from build123d import *

# Parameters (mm, degrees)
SKETCH1_R           = 107.09
BOSS_EXTRUDE1_DEPTH = 3
CUT_EXTRUDE1_START  = -3
CUT_EXTRUDE1_DEPTH  = 4
CIRPATTERN1_COUNT   = 8
SKETCH7_W           = 3
SKETCH7_H           = 5
CUT_EXTRUDE4_DEPTH  = 3
CIRPATTERN2_COUNT   = 8
SKETCH4_R           = 1.5
SKETCH4_W           = 66
SKETCH4_H           = 30
CUT_EXTRUDE5_DEPTH  = 10
CUT_EXTRUDE6_DEPTH  = 3


with BuildPart() as part:
    # Sketch1 → Boss-Extrude1 (new body)
    with BuildSketch(Plane(origin=(0, 0, 0), x_dir=(1, 0, 0), z_dir=(0, 1, 0))):
        Circle(SKETCH1_R)
    extrude(amount=BOSS_EXTRUDE1_DEPTH)

    # Sketch2 → Cut-Extrude1 (cut)
    with BuildSketch(Plane(origin=(0, 3, 0), x_dir=(1, 0, 0), z_dir=(0, 1, 0)).offset(CUT_EXTRUDE1_START)):
        Polygon((-1.5, 597.330930071), (-1.5, 107.079494302), (-1.5, 97.079494302), (1.5, 97.079494302), (1.5, 107.079494302), (1.5, 597.330930071), (1.5, 1577.83380161), (-1.5, 1577.83380161), align=None)
    cut_extrude1 = extrude(amount=CUT_EXTRUDE1_DEPTH, mode=Mode.SUBTRACT)

    # CirPattern1: Cut-Extrude1 ×8 about axis
    cirpattern1_axis = Axis((0, 0, 0), (0, -1, 0))
    for i in range(1, CIRPATTERN1_COUNT):
        add(cut_extrude1.rotate(cirpattern1_axis, i * 360 / CIRPATTERN1_COUNT), mode=Mode.SUBTRACT)

    # Sketch7 → Cut-Extrude4 (cut)
    with BuildSketch(Plane(origin=(0, 3, 0), x_dir=(1, 0, 0), z_dir=(0, 1, 0))):
        with Locations((-3.5, 93.579494302)):
            Rectangle(SKETCH7_W, SKETCH7_H)
        with Locations((3.5, 93.579494302)):
            Rectangle(SKETCH7_W, SKETCH7_H)
    cut_extrude4 = extrude(amount=-CUT_EXTRUDE4_DEPTH, mode=Mode.SUBTRACT)

    # CirPattern2: Cut-Extrude4 ×8 about axis
    cirpattern2_axis = Axis((0, 0, 0), (0, 1, 0))
    for i in range(1, CIRPATTERN2_COUNT):
        add(cut_extrude4.rotate(cirpattern2_axis, i * 360 / CIRPATTERN2_COUNT), mode=Mode.SUBTRACT)

    # Sketch4 → Cut-Extrude5 (cut)
    with BuildSketch(Plane(origin=(0, 3, 0), x_dir=(1, 0, 0), z_dir=(0, 1, 0))):
        with Locations((-57, 9.5)):
            Circle(SKETCH4_R)
        with Locations((-57, -9.5)):
            Circle(SKETCH4_R)
        with Locations((21, -9.5)):
            Circle(SKETCH4_R)
        with Locations((21, 9.5)):
            Circle(SKETCH4_R)
        with Locations((-18, 0)):
            Rectangle(SKETCH4_W, SKETCH4_H)
        with BuildLine():
            Line((72.75038213, -25.5), (-72.75038213, -25.5))
            ThreePointArc((-72.75038213, -25.5), (0, -77.09), (72.75038213, -25.5))
        make_face()
        with BuildLine():
            Line((72.75038213, 25.5), (-72.75038213, 25.5))
            ThreePointArc((-72.75038213, 25.5), (0, 77.09), (72.75038213, 25.5))
        make_face()
    extrude(amount=-CUT_EXTRUDE5_DEPTH, mode=Mode.SUBTRACT)

    # Sketch9 → Cut-Extrude6 (cut)
    with BuildSketch(Plane(origin=(0, 3, 0), x_dir=(1, 0, 0), z_dir=(0, 1, 0))):
        Polygon((-35.879388071, -94.459883081), (-33.107749474, -95.607933378), (-26.219447691, -78.978101793), (-28.991086289, -77.830051496), align=None)
        Polygon((-19.249556486, -101.348184863), (-16.477917889, -102.49623516), (-9.589616106, -85.866403575), (-12.361254704, -84.718353278), align=None)
        Polygon((53.935833667, 67.497598822), (60.824135449, 84.127430407), (58.052496852, 85.275480704), (51.164195069, 68.645649119), align=None)
        Polygon((37.306002081, 74.385900604), (44.194303864, 91.015732189), (41.422665266, 92.163782487), (34.534363484, 75.533950901), align=None)
    extrude(amount=-CUT_EXTRUDE6_DEPTH, mode=Mode.SUBTRACT)


solid = part.part
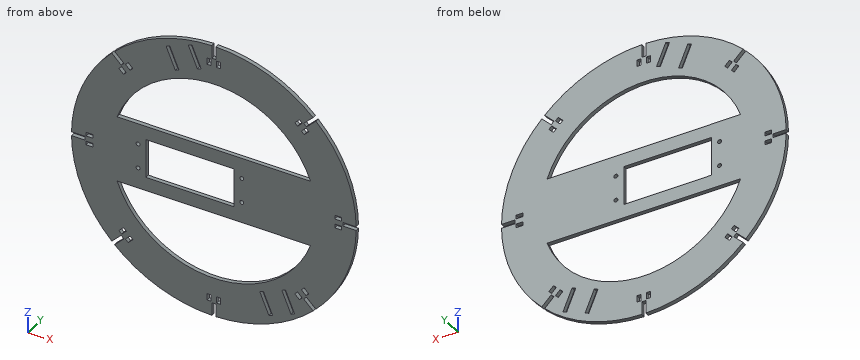
Could you check a few things on this model? Use its own coordinates, in mm. Coordinates: 2 decimals unless noted, no trailing zeros. Write each loop counter-clockwise with the first axis right and the second up, starting at its lowest first coordinate (ties: lowest second). Pieces come first, ordered by that corner, then holes. Notation, with made-up numbers: (74.5, 74.25) - (93.5, 74.25) arc R24 cw to (93.5, 90.25) - close; hole circle Ø9 at (30.5, 25). An arc over 180 degrees is marked (long way). Write item = value, one per line.
1) Suppose I cut it at A-A on x = 48. Please give me the cut outline in (y, z), plus the area to 3 significant figures.
Result set:
outline = (0, -95.73) - (3, -95.73) - (3, -60.32) - (0, -60.32) - close; (0, -25.5) - (3, -25.5) - (3, 25.5) - (0, 25.5) - close; (0, 60.32) - (3, 60.32) - (3, 95.73) - (0, 95.73) - close
area = 365 mm2
2) Suppose I cut it at C-C on y = 2.4. State how many separate pieces and enclosed holes the cut face has, plus the area to 3 significant figures.
Result set:
separate_pieces = 1
enclosed_holes = 27
area = 22,400 mm2
3) Please list where these lines run through material, in increasing order: line 1 (X direction, y = 1.2, z = 4.5); line 2 (Z direction, x = -33.5, y = 0.65); line 3 (X direction, y = 2.25, z = 68.5). Write a range as [from, to].
Result set:
line_1 = [-107, -96.08], [-91.08, -51], [15, 91.08], [96.08, 107]
line_2 = [-101.72, -69.43], [-25.5, -15], [15, 25.5], [69.43, 88.72], [95.45, 101.72]
line_3 = [-82.32, -70.62], [-68.79, -65.67], [-61.43, -35.36], [35.36, 61.43], [65.67, 68.79], [70.62, 82.32]
4) Suppose I cut it at B-B on z = 44.5. Please give me the cut outline in (x, y), plus the area to 3 significant figures.
Result set:
outline = (-97.41, 0) - (-62.95, 0) - (-62.95, 3) - (-97.41, 3) - close; (62.95, 0) - (97.41, 0) - (97.41, 3) - (62.95, 3) - close
area = 207 mm2
5) Suppose I cut it at D-D on z = 21. Please give me the cut outline in (x, y).
Result set:
outline = (-105.01, 0) - (105.01, 0) - (105.01, 3) - (-105.01, 3) - close
6) Will these pins go through, and if not, where does the flat tip stop? pin 1 Ø1.5 at (y, z) = (1.5, -0.5) entering from +X; pin 2 Ø1.5 at (x, y) = (94.5, 2) entering from -Z; pin 3 Ø1.5 at (x, y) = (4, 2) entering from -Z.
Result set:
pin_1 = 97.08
pin_2 = -51.76
pin_3 = -107.04
